CAD build for the part. Positions are in the model's coordinates, mm. A direction names the side the tool comes from. Round coordinates to 2 decimals unless told otherwise and drop trailing zeros. Loops run counter-clockwise (first coordinate to the right, second up) from the corner with the lowest first, then second, coordinate; pieces in that order, holes last. Notation, with made-up numbers: (-32, -30.5) - (-19, -30.5) arc R15 cw to (-19, -24.5) - close; hole circle Ø10 at (1, -24.5). An arc over 180 degrees is marked (long way). One line per question, with ' | ' between items.
```python
from build123d import *

# Parameters (mm, degrees)
F0_W        = 11.43
F0_H        = 11.43
F0_R        = 2.15265
F1_DEPTH    = 22.4125
F2_W        = 11.43
F2_H        = 11.43
F3_DEPTH    = 1.5875
F4_R        = 1.35255
F5_REACH    = 15.2565891076
F6_T1_DEPTH = 52.575
F7_R        = 2.15265
F8_DEPTH    = 60.325


# Not quite as in the source:
# - a fillet or chamfer that OpenCascade refuses, or shapes differently, is made with other operations: its cross-section is extruded or revolved along the edge and cut away or added


with BuildPart() as f1:
    # F0 (on Top) → F1 (new body)
    with BuildSketch(Plane.XY):
        Rectangle(F0_W, F0_H)
        Circle(F0_R, mode=Mode.SUBTRACT)
    extrude(amount=F1_DEPTH)

    # F2 (on face) → F3 (join)
    with BuildSketch(Plane.XY.offset(22.4125)):
        Rectangle(F2_W, F2_H)
    extrude(amount=F3_DEPTH)

    f5_end = f1.faces().sort_by_distance((-2.15265, 0, 11.20625))[0]
    # F4 (on face) → F5 (cut, up to a face of the model that its end follows)
    with BuildSketch(Plane(origin=(-5.715, 0, 0), x_dir=(0, -1, 0), z_dir=(-1, 0, 0))):
        with Locations((0, 11.20625)):
            Circle(F4_R)
    f5_long = extrude(amount=-F5_REACH, mode=Mode.PRIVATE)
    add(split(f5_long, bisect_by=f5_end, keep=Keep.ALL, mode=Mode.PRIVATE).solids().sort_by_distance((-5.715, 0, 11.20625))[0], mode=Mode.SUBTRACT)

    # F6: fillet of radius 5.715 on 4 edges, made by hand

    # F6_s2 → F6_t1 (cut)
    with BuildSketch(Plane.XY.offset(-14.2875)):
        with BuildLine():
            ThreePointArc((0, -5.715), (-4.0411152545, -4.0411152545), (-5.715, 0))
            Line((-5.715, 0), (-5.715, -5.715))
            Line((-5.715, -5.715), (0, -5.715))
        make_face()
        with BuildLine():
            ThreePointArc((0, -5.715), (4.0411152545, -4.0411152545), (5.715, 0))
            Line((5.715, 0), (5.715, -5.715))
            Line((5.715, -5.715), (0, -5.715))
        make_face()
        with BuildLine():
            ThreePointArc((-5.715, 0), (-4.0411152545, 4.0411152545), (0, 5.715))
            Line((0, 5.715), (-5.715, 5.715))
            Line((-5.715, 5.715), (-5.715, 0))
        make_face()
        with BuildLine():
            ThreePointArc((5.715, 0), (4.0411152545, 4.0411152545), (0, 5.715))
            Line((0, 5.715), (5.715, 5.715))
            Line((5.715, 5.715), (5.715, 0))
        make_face()
    extrude(amount=F6_T1_DEPTH, mode=Mode.SUBTRACT)

    # F7 (on face) → F8 (join)
    with BuildSketch(Plane.XY.offset(24)):
        Circle(F7_R)
    extrude(amount=F8_DEPTH)


solid = f1.part
```
(1) Cut at D-D, the plane x = 3.75. Write the cut outline in (y, z).
Results found:
outline: (-4.31, 0) - (4.31, 0) - (4.31, 24) - (-4.31, 24) - close
(2) Tool access for faces 4 (the face through (2.053, 0.647, 11.049)), 5 (the face through (-3.72, 1.35, 11.27)), 6 (the face through (-0.1, -2.5, 24)): list every direction of +Z, -Z, +X, -X, +Y, -Y with a clear straight run to the whole face (end or side of a thin tool).
Results found:
face 4: -Z | face 5: -X | face 6: +Z
(3) Drop a flat-ended pin along its axis: P1, Ø1.5, axis at y = -2, z = 55, coming from the +X side. Give the stop position or say it passes through.
Results found:
P1: stops at x = 1.75
(4) Two-plate mould, pull along Y, no slides. Class faces 1 (the face through (0, 0, 84.325)), 2 (the face through (0, 0, 22.412)), 3 (the face through (-0.28, 2.134, 53.74)): released by +Y, released by -Y, zero draft, split by the parting line, or undercut.
Results found:
face 1: zero draft | face 2: undercut | face 3: split by the parting line
(5) Probe L1, parallel to X at y = 0, z = 13.5 (3 decimals); L2, parallel to Z at x = -3.95, y = 0. List the from-to ranges inside material, lowest first.
Results found:
L1: x = -5.715 to -2.153, 2.153 to 5.715 | L2: z = 0 to 9.85, 12.56 to 24
(6) Cut at A-A, the plane z = 9. Write the cut outline in (x, y) (3 decimals), then the cut area to 3 significant figures.
Results found:
outline: circle Ø11.43 at (0, 0); hole circle Ø4.305 at (0, 0) | area: 88.1 mm²
(7) Cut at C-C, the plane y = -3. Write the cut outline in (x, z), then the cut area to 3 significant figures.
Results found:
outline: (-4.86, 0) - (4.86, 0) - (4.86, 24) - (-4.86, 24) - close | area: 233 mm²
(8) Cut at B-B, the plane z = 64.5. Write the cut outline in (x, y).
Results found:
outline: circle Ø4.31 at (0, 0)
